For this review, take the finished solid that the model builds, in its own axes (mm). Give positions to 0.01 mm unless a question says otherwise; leave off trailing zeros. Write each loop counter-clockwise with the first axis right and the second up, starting at its lowest first coordinate (ties: lowest second). Pieces come first, ordered by that corner, then holes. Notation, with made-up numbers: (78, 44) -> (136, 44) arc R20 cw to (136, 69) -> close; hole circle Ø10 at (31, 72.5). An arc over 180 degrees is marked (long way). Return JSON: item names as keys, results as strings.
Autodesk Inventor part; units mm, degrees
ref_plane "YZ Plane" through (0, 0, 0) normal (1, 0, 0) x (0, 1, 0)
ref_plane "XZ Plane" through (0, 0, 0) normal (0, 1, 0) x (-1, 0, 0)
ref_plane "XY Plane" through (0, 0, 0) normal (0, 0, 1) x (1, 0, 0)
sketch "Sketch1" plane through (0, 0, 0) normal (0, 0, 1) x (1, 0, 0)
  line L0 (51.9615, 90) -> (103.923, 0)
  line L1 (103.923, 0) -> (51.9615, -90)
  line L2 (51.9615, -90) -> (-51.9615, -90)
  line L3 (-51.9615, -90) -> (-103.923, 0)
  line L4 (-103.923, 0) -> (-51.9615, 90)
  line L5 (-51.9615, 90) -> (51.9615, 90)
  circle A0 centre (0, 0) radius 10
  dimension "d3" = 180
  dimension "d13" = 20
extrude "Extrusion1" add sketch "Sketch1" along normal blind 4.7625
sketch "Sketch2" plane through (0, 0, 0) normal (0, 0, -1) x (-1, 0, 0)
  line L0 (-51.9615, 90) -> (-103.923, 0)
  line L1 (51.9615, -90) -> (103.923, 0)
  line L2 (103.923, 0) -> (51.9615, 90)
  line L3 (51.9615, 90) -> (-51.9615, 90)
  line L4 (-51.9615, 90) -> (0, 180) construction
  line L5 (0, 180) -> (51.9615, 90) construction
  arc A0 (-68.5, 61.3545) -> (-61, 74.3449) centre (-64.75, 67.8497) ccw
  arc A1 (-46.6506, 90) -> (-54.617, 85.4006) centre (-46.6506, 80.8013) ccw
  arc A2 (-94.8846, 15.6551) -> (-87.3846, 28.6455) centre (-91.1346, 22.1503) ccw
  line L6 (-103.923, 0) -> (-155.8846, -90) construction
  line L7 (-155.8846, -90) -> (-51.9615, -90) construction
  line L8 (-103.923, 0) -> (-51.9615, -90)
  arc A3 (-101.2676, 4.5994) -> (-101.2676, -4.5994) centre (-93.3013, 0) ccw
  point P0 (0, 0)
  dimension "d5" = 7.5
  dimension "d6" = 129.5
  dimension "d7" = 9.1987
  dimension "d8" = 93.3013
  dimension "d9" = 129.5
extrude "Extrusion2" cut sketch "Sketch2" against normal up to next
pattern_circular "Circular Pattern1" count 3 over 360 about axis through (0, 0, 0) along (0, 0, 1) of "Extrusion2"
fillet "Fillet1" radius 5 12 edges at (61, 74.3449, 2.3813) (68.5, 61.3545, 2.3813) (87.3846, 28.6455, 2.3813) (94.8846, 15.6551, 2.3813) (-68.5, 61.3545, 2.3813) (-61, 74.3449, 2.3813) (-94.8846, 15.6551, 2.3813) (-87.3846, 28.6455, 2.3813) (-18.8846, -90, 2.3813) (-33.8846, -90, 2.3813) (33.8846, -90, 2.3813) (18.8846, -90, 2.3813)
equation "\"d9\" = d6"
properties part number "Heatbed_Insulator_Cork" material "Cork Tiles"
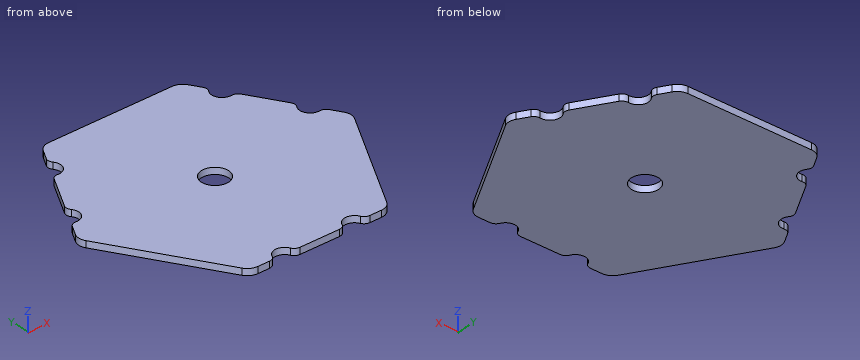
1. Add section C-C, the plane y = 21. State the section outline as (x, z) points.
Results found:
{"outline": "(-83.72, 0) -> (83.72, 0) -> (83.72, 4.76) -> (-83.72, 4.76) -> close"}
2. Add section B-B, the plane x = 0. State the section outline as (y, z) points.
Results found:
{"outline": "(-90, 0) -> (-10, 0) -> (-10, 4.76) -> (-90, 4.76) -> close; (10, 0) -> (90, 0) -> (90, 4.76) -> (10, 4.76) -> close"}
3. For pin 1 (2 mm diameter, centred on x = -49, z = 1, fed in from +Y); pin 2 (1 mm diameter, centred on x = -20, z = 3.5, fed in from -Y); pin 3 (2 mm diameter, centred on x = 36, z = 1.5, fed in from -Y), all flat-tipped, find the tip position at first contact; note any pin that passes through.
Results found:
{"pin 1": "stops at y = 89.9", "pin 2": "stops at y = -87.02", "pin 3": "stops at y = -89.93"}
4. Add section A-A, the plane y = 0. State the section outline as (x, z) points.
Results found:
{"outline": "(-102.5, 0) -> (-10, 0) -> (-10, 4.76) -> (-102.5, 4.76) -> close; (10, 0) -> (102.5, 0) -> (102.5, 4.76) -> (10, 4.76) -> close"}
5. To check wall thickness, follow probe 1 along Y at (x, z) = (0, 3.2); probe 2 along X at (y, z) = (55, 3.1); probe 3 along X at (y, z) = (53, 2.9). State the ranges of each line that lie inside material, in increasing order.
Results found:
{"probe 1": "y = -90 to -10, 10 to 90", "probe 2": "x = -72.17 to 72.17", "probe 3": "x = -73.32 to 73.32"}
